Verification items for the finished model (mm, model axes). Face numbers are marked on the shaded views. A direction names the side the tool comes from. Coordinates: 2 decimals unless noted, no trailing zeros. Loops run counter-clockwise (first coordinate to the right, second up) from the corner with the lowest first, then second, coordinate; pieces in that order, holes last. Notation, with made-up numbers: (23.5, 61) -> (66.5, 61) arc R19 ccw to (66.5, 68) -> close; hole circle Ø10 at (57, 24). An arc over 180 degrees is marked (long way). Answer as a JSON object with one key per item and string values. Group by question number.
Q1. Set-up check for the marked faces 1 and 2: record each of +Z, -Z, +X, -X, +Y, -Y from which the full face is reachable in a straight line by a thin tool's end or side.
Q2. Cross-section at A-A on x = 80. Record the boundary of the cut face in (y, z) (3 decimals), and give its area (3 significant figures).
Q3. Gauge pin test, flat end, axial feed: pin 1 Ø10.5 at (x, z) = (80, 20) entering from -Y. Record the tip position at first contact, or that the pin passes through.
Q4. Scan lines: L1, parallel to Z at x = 25, y = -33.25; L2, parallel to X at y = -38.5, z = 23.5; L3, parallel to X at y = -33, z = 10. Record each from-to range of solid material in increasing order.
Q5. Release check for a two-part mould opening along Z. For the marked faces 3, 4, 5 and 6 record: released by +Z, released by -Z, zero draft, split by the parting line, or undercut.
Q6. Cross-section at B-B on y = -9. Record the boundary of the cut face in (x, z).
Q7. Cross-section at D-D on y = -36. Record the boundary of the cut face in (x, z) (3 decimals), and give its area (3 significant figures).
Q8. Cross-section at C-C on z = 20. Record the boundary of the cut face in (x, y) (3 decimals).
```python
from build123d import *

# Parameters (mm, degrees)
F0_W           = 90
F0_H           = 40
F1_DEPTH       = 41
F3_D           = 8.5
F3_CBORE_D     = 17.25
F3_CBORE_DEPTH = 10
F4_D           = 6.8
F4_DEPTH       = 18.25
F4_TIP         = 2.0429261047


with BuildPart() as f1:
    # F0 (on Front) → F1 (new body)
    with BuildSketch(Plane.XZ):
        with Locations((45, 20)):
            Rectangle(F0_W, F0_H)
    extrude(amount=F1_DEPTH)

    # F3 (through all)
    with Locations(Plane.XZ.offset(41)):
        with Locations((10, 20), (80, 20)):
            CounterBoreHole(F3_D / 2, F3_CBORE_D / 2, F3_CBORE_DEPTH)

    # F4
    with Locations(Plane.XZ.offset(41)):
        with Locations((25, 30), (65, 10)):
            Hole(F4_D / 2, depth=F4_DEPTH)
            with Locations((0, 0, -(F4_DEPTH + F4_TIP / 2))):  # 118° drill point
                Cone(0, F4_D / 2, F4_TIP, mode=Mode.SUBTRACT)


solid = f1.part
```
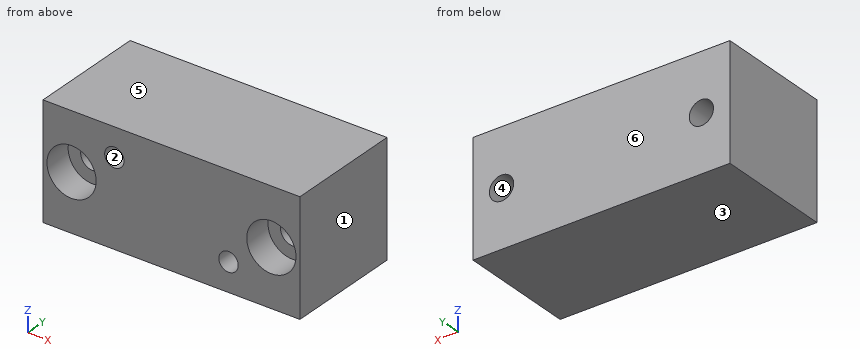
Computed values:
{
 "1": {"face 1": "+Z, -Z, +X, +Y, -Y", "face 2": "-Y"},
 "2": {"outline": "(-41, 0) -> (0, 0) -> (0, 15.75) -> (-31, 15.75) -> (-31, 11.375) -> (-41, 11.375) -> close; (-41, 28.625) -> (-31, 28.625) -> (-31, 24.25) -> (0, 24.25) -> (0, 40) -> (-41, 40) -> close", "area": "1,200 mm²"},
 "3": {"pin 1": "stops at y = -31"},
 "4": {"L1": "z = 0 to 26.6, 33.4 to 40", "L2": "x = 0 to 2.12, 17.88 to 72.12, 87.88 to 90", "L3": "x = 0 to 61.6, 68.4 to 90"},
 "5": {"face 3": "released by -Z", "face 4": "undercut", "face 5": "released by +Z", "face 6": "zero draft"},
 "6": {"outline": "(0, 0) -> (90, 0) -> (90, 40) -> (0, 40) -> close; hole circle Ø8.5 at (10, 20); hole circle Ø8.5 at (80, 20)"},
 "7": {"outline": "(0, 0) -> (90, 0) -> (90, 40) -> (0, 40) -> close; hole circle Ø17.25 at (10, 20); hole circle Ø6.8 at (25, 30); hole circle Ø6.8 at (65, 10); hole circle Ø17.25 at (80, 20)", "area": "3,060 mm²"},
 "8": {"outline": "(0, -41) -> (1.375, -41) -> (1.375, -31) -> (5.75, -31) -> (5.75, 0) -> (0, 0) -> close; (14.25, -31) -> (18.625, -31) -> (18.625, -41) -> (71.375, -41) -> (71.375, -31) -> (75.75, -31) -> (75.75, 0) -> (14.25, 0) -> close; (84.25, -31) -> (88.625, -31) -> (88.625, -41) -> (90, -41) -> (90, 0) -> (84.25, 0) -> close"}
}
